Read the model definition and answer for the solid it produces. Units are mm, in the model's axes. Coordinates: 2 decimals unless noted, no trailing zeros. Loops run counter-clockwise (first coordinate to the right, second up) from the corner with the lowest first, then second, coordinate; pieces in that order, holes last. Notation, with made-up numbers: (71, 41.5) -> (119, 41.5) arc R32 cw to (119, 69.5) -> close; hole circle Ø10 at (21.25, 14). An arc over 180 degrees is marked (long way). Answer as a JSON object with one key per item and string values. Group by question number.
1) Section B-B, the plane z = -38.1 is taken. Give the vertices of the cut face in (x, y).
2) A flat-ended cylindrical pin translates along its axis: P1, Ø3, axis at x = 3.175, z = -73.025, coming from the +Y side. Find the tip coordinate at first contact, or state that the pin passes through.
3) Consider probe 1 along Z at (x, y) = (38, 0.6); probe 2 along X at (y, z) = (1, -38.5); probe 3 along X at (y, z) = (2.4, -36.5). Determine where each line is inside the solid, lowest interval first. Write a range as [from, to].
4) Section A-A, the plane x = 38.1 is taken. Give the vertices of the cut face in (y, z).
Autodesk Inventor part; units mm, degrees
ref_plane "YZ Plane" through (0, 0, 0) normal (1, 0, 0) x (0, 1, 0)
ref_plane "XZ Plane" through (0, 0, 0) normal (0, 1, 0) x (-1, 0, 0)
ref_plane "XY Plane" through (0, 0, 0) normal (0, 0, 1) x (1, 0, 0)
sketch "Sketch1" plane through (0, 0, 0) normal (0, 1, 0) x (-1, 0, 0)
  line L0 (0, 0) -> (-76.2, 0)
  line L1 (-76.2, 0) -> (-76.2, -76.2)
  line L2 (-76.2, -76.2) -> (0, -76.2)
  line L3 (0, -76.2) -> (0, 0)
  line L4 (-38.1, -76.2) -> (-38.1, -73.025)
  circle A0 centre (-38.1, -73.025) radius 2.1844
  line L5 (0, -38.1) -> (-3.175, -38.1)
  line L6 (-38.1, 0) -> (-38.1, -3.175)
  line L7 (-76.2, -38.1) -> (-73.025, -38.1)
  circle A1 centre (-3.175, -38.1) radius 2.1844
  circle A2 centre (-73.025, -38.1) radius 2.1844
  circle A3 centre (-38.1, -3.175) radius 2.1844
  circle A4 centre (-3.175, -73.025) radius 1.778
  circle A5 centre (-3.175, -3.175) radius 1.778
  circle A6 centre (-73.025, -3.175) radius 1.778
  circle A7 centre (-73.025, -73.025) radius 1.778
  dimension "d0" = 76.2
  dimension "d1" = 76.2
  dimension "d2" = 3.175
  dimension "d3" = 4.3688
  dimension "d4" = 3.175
  dimension "d5" = 3.175
  dimension "d6" = 3.175
  dimension "d7" = 4.3688
  dimension "d8" = 4.3688
  dimension "d9" = 4.3688
  dimension "d10" = 3.556
  dimension "d11" = 3.556
  dimension "d12" = 3.556
  dimension "d13" = 3.556
extrude "Extrusion1" add sketch "Sketch1" along normal blind 3.302
sketch "Sketch2" plane through (0, 0, 0) normal (0, 0, 1) x (1, 0, 0)
  line L0 (76.2, 0) -> (76.2, 3.302)
  circle A0 centre (50.8, 1.651) radius 0.508
  point P0 (0, 0)
  dimension "d17" = 1.016
extrude "Extrusion2" cut sketch "Sketch2" against normal blind 12.7
properties part number "cold_plate"
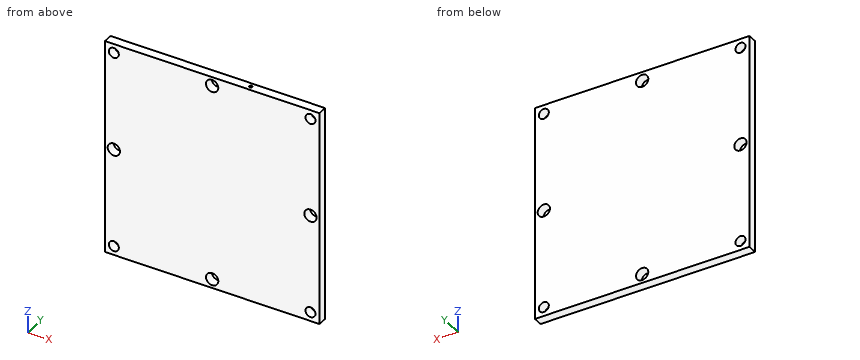
Determined:
{
 "1": {"outline": "(0, 0) -> (0.99, 0) -> (0.99, 3.3) -> (0, 3.3) -> close; (5.36, 0) -> (70.84, 0) -> (70.84, 3.3) -> (5.36, 3.3) -> close; (75.21, 0) -> (76.2, 0) -> (76.2, 3.3) -> (75.21, 3.3) -> close"},
 "2": {"P1": "through"},
 "3": {"probe 1": "[-76.2, -75.21], [-70.84, -5.36], [-0.99, 0]", "probe 2": "[0, 1.03], [5.32, 70.88], [75.17, 76.2]", "probe 3": "[0, 1.69], [4.66, 71.54], [74.51, 76.2]"},
 "4": {"outline": "(0, -76.2) -> (3.3, -76.2) -> (3.3, -75.21) -> (0, -75.21) -> close; (0, -70.84) -> (3.3, -70.84) -> (3.3, -5.36) -> (0, -5.36) -> close; (0, -0.99) -> (3.3, -0.99) -> (3.3, 0) -> (0, 0) -> close"}
}
